Verification items for this drawing (mm, ordinates from the low corner). A direction names the side the tool comes from. Round coordinates to 2 decimals unless told otherwise and drop trailing zeros. Loops run counter-clockwise (first coordinate to the right, second up) from the corner with the lowest first, then second, coordinate; pieces in that order, holes last. Notation, with made-up numbers: (-16.5, -21.5) - (24.5, -21.5) arc R23 ccw to (24.5, 16.5) - close; hole circle Ø3 at (61.25, 3). An arc over 180 degrees is marked (long way). Put each result on its own line as item: value.
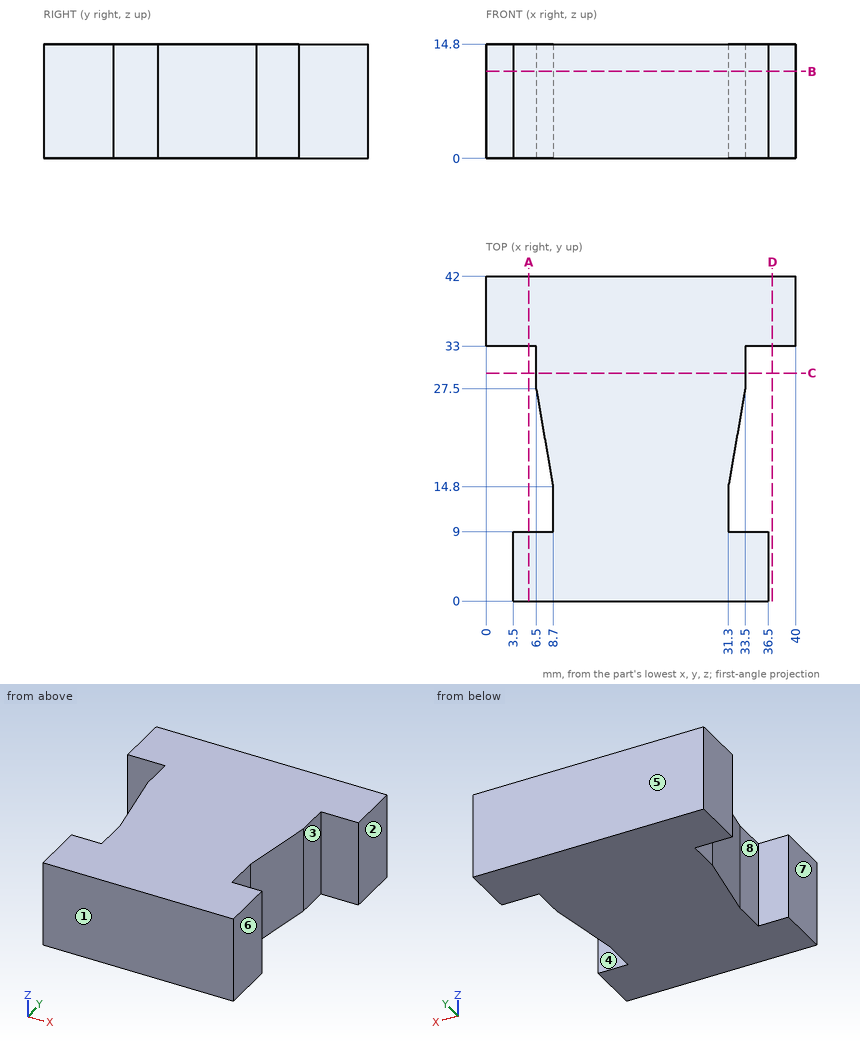
Item 1: Section check D-D on x = 37. Enter the section's corners in (y, z).
Filled sheet:
outline: (33, 0) - (42, 0) - (42, 14.8) - (33, 14.8) - close
Item 2: Section check A-A on x = 5.5. Enter the section's corners in (y, z), then the cut area to 3 significant figures.
Filled sheet:
outline: (0, 0) - (9, 0) - (9, 14.8) - (0, 14.8) - close; (33, 0) - (42, 0) - (42, 14.8) - (33, 14.8) - close
area: 266 mm²
Item 3: Release check for a two-part mould opening along Y. For the marked faces 1, 2 and 3 record: +Y half, -Y half, draft (parallel to the pull), parting line (faces both ways), or undercut.
Filled sheet:
face 1: -Y half
face 2: draft
face 3: undercut
Item 4: Thickness scan on line 1 (X direction, y = 14, z = 6); line 2 (X direction, y = 28.5, z = 10). Record the ranges inside material, lowest first. Write a range as from..to.
Filled sheet:
line 1: 8.7..31.3
line 2: 6.5..33.5
Item 5: Section check B-B on z = 11.25. Enter the section's corners in (x, y), then the cut area to 3 significant figures.
Filled sheet:
outline: (0, 33) - (6.5, 33) - (6.5, 27.5) - (8.7, 14.8) - (8.7, 9) - (3.5, 9) - (3.5, 0) - (36.5, 0) - (36.5, 9) - (31.3, 9) - (31.3, 14.8) - (33.5, 27.5) - (33.5, 33) - (40, 33) - (40, 42) - (0, 42) - close
area: 1,250 mm²
Item 6: Go/stop test with flat-tipped pins: pin 1 (2.5 mm diameter, centred on y = 4, z = 5, fed in from -X); pin 2 (1.7 mm diameter, centred on y = 11, z = 10.5, fed in from -X); pin 3 (6.5 mm diameter, centred on y = 12.5, z = 4.5, fed in from +X). Record where each tip stops, or that it passes through.
Filled sheet:
pin 1: x = 3.5
pin 2: x = 8.7
pin 3: x = 31.46
Item 7: Section check C-C on y = 29.5. Enter the section's corners in (x, z), then the cut area to 3 significant figures.
Filled sheet:
outline: (6.5, 0) - (33.5, 0) - (33.5, 14.8) - (6.5, 14.8) - close
area: 400 mm²
Item 8: Tool access check on the marked faces 4, 5, 6, 7 and 8. Record the directions out of +Z, -Z, +X, -X, +Y, -Y that give a thin tool (end or side, any length) a straight path to the whole face; none if there is none.
Filled sheet:
face 4: +Z, -Z, +X
face 5: +Z, -Z, +X, -X, +Y
face 6: +Z, -Z, +X, -Y
face 7: +Z, -Z, -X, -Y
face 8: +Z, -Z, -X
